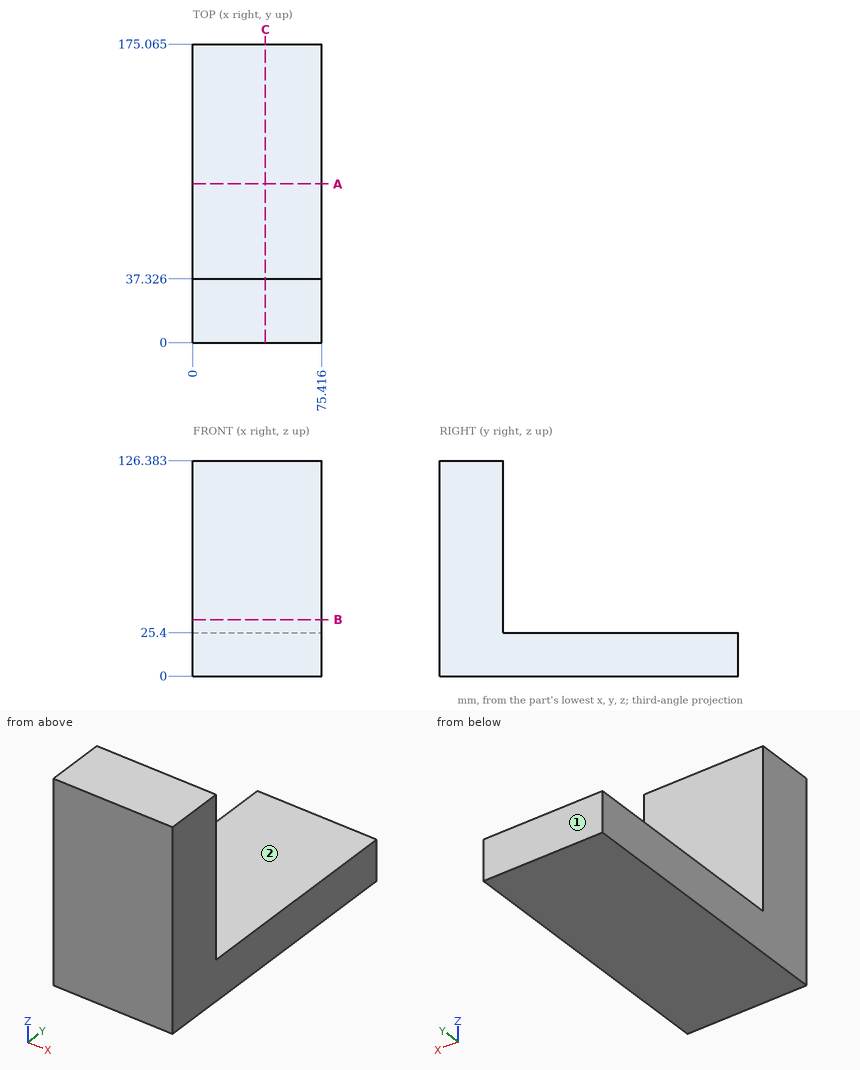
Study the drawing (mm; zero at the part's minimum x, y, z) and answer. A direction names the side the tool comes from. Give positions to 0.01 mm unless a question says otherwise; leave off trailing zeros. Loops run counter-clockwise (first coordinate to the right, second up) from the corner with the lowest first, then second, coordinate; pieces in that order, holes last. Notation, with made-up numbers: (33.5, 10) - (80.5, 10) arc R23 cw to (80.5, 23) - close; hole circle Ø6 at (21.5, 67). An arc over 180 degrees is marked (long way). Return JSON: item names as keys, results as strings. Group by question number.
1. Straight lines are drawn through the part: line 1 (Y direction, x = 13, z = 34); line 2 (Z direction, x = 39, y = 132). For each, find the intervals that lie inside material, in ascending order. Write a range as [from, to].
2. Which of the six approach directions +Z, -Z, +X, -X, +Y, -Y give full straight-line access (tool end or side, diameter ignored) to the marked faces 1 and 2?
3. Find section A-A (y = 93). Write down the section's boundary in (x, z), then the cut area to 3 significant figures.
4. Find section B-B (z = 33). Write down the section's boundary in (x, y).
5. Find section C-C (x = 42.5). Write down the section's boundary in (y, z) (1 decimal).
6. Given pin 1 Ø10 at (x, y) = (23, 139) entering from -Z; pin 2 Ø3 at (x, y) = (27.5, 57.5) entering from +Z, each flat-ended and moving along its own axis, determine where each tip first touches the part or whether it passes through.
Verdict:
{
 "1": {"line 1": "y = [0, 37.33]", "line 2": "z = [0, 25.4]"},
 "2": {"face 1": "+Z, -Z, +X, -X, +Y", "face 2": "+Z, +X, -X, +Y"},
 "3": {"outline": "(0, 0) - (75.42, 0) - (75.42, 25.4) - (0, 25.4) - close", "area": "1,920 mm^2"},
 "4": {"outline": "(0, 0) - (75.42, 0) - (75.42, 37.33) - (0, 37.33) - close"},
 "5": {"outline": "(0, 0) - (175.1, 0) - (175.1, 25.4) - (37.3, 25.4) - (37.3, 126.4) - (0, 126.4) - close"},
 "6": {"pin 1": "stops at z = 0", "pin 2": "stops at z = 25.4"}
}
